Geometry: final body of the model. Coordinates: model frame, mm. Face numbers are marked on the shaded views. A direction names the side the tool comes from. Coordinates: 2 decimals unless noted, no trailing zeros. Write each loop counter-clockwise with the first axis right and the second up, starting at its lowest first coordinate (ties: lowest second). Pieces come first, ordered by that corner, then holes. Notation, with made-up numbers: M 60.25,29 L 68.25,29 A16 ccw 68.25,42 Z; hole C 22,81 d9. An arc over 180 degrees is marked long. Write item = value, one per line. Start each with the question number.
Item 1: First-contact query: pin 1 Ø5 at (y, z) = (6.5, 10.5) entering from +X; pin 2 Ø0.9 at (y, z) = (6.5, 13) entering from +X; pin 3 Ø3 at (y, z) = (5.5, 13.5) entering from -X. Flat tips, straight axial feed; report the tip coordinate or a pass-through.
Item 2: Section A-A on x = 0. Output: boundary loops of the cut face in (y, z).
Item 3: Section D-D on x = -6. Output: boundary loops of the cut face in (y, z).
Item 4: Reachability of the marked faces 5, 6, 7 and 8 from +Z, -Z, +X, -X, +Y, -Y: full face, straight path, thin tool, end or side. Return the list, or none.
Item 5: Ray query, L1, parallel to Z at x = 0, y = 3.5; L2, parallel to X at y = 1.25, z = -10; L3, parallel to X at y = 4.75, z = 6.75. Return the intervals inside material, ascending. Write a range as [from, to].
Item 6: Pull-direction query (Z, two-part tool) for the marked faces 1, 2, 3 and 4; classes: +Z half, -Z half, draft (parallel to the pull), parting line (faces both ways), or undercut.
Item 7: Section B-B on z = 13.25. Output: boundary loops of the cut face in (x, y).
Item 8: Section C-C on z = -5. Output: boundary loops of the cut face in (x, y), plus the area to 3 significant figures.
Autodesk Inventor part; units mm, degrees
ref_plane "Work Plane1" through (0, 10, 0) normal (0, 1, 0) x (-1, 0, 0)
ref_plane "XY Plane" through (0, 0, 0) normal (0, 0, 1) x (1, 0, 0)
sketch "Sketch1" plane through (0, 0, 0) normal (0, 1, 0) x (-1, 0, 0)
  circle A0 centre (0, 0) radius 15
  dimension "d0" = 30
ref_plane "Work Plane1" through (0, 10, 0) normal (0, 1, 0) x (-1, 0, 0)
extrude "Extrusion1" add sketch "Sketch1" along normal blind 10
sketch "Sketch2" plane through (0, 10, 0) normal (0, 1, 0) x (1, 0, 0)
  line L0 (2, -22) -> (-2, -22)
  line L1 (-2, -22) -> (-2, -12)
  line L2 (-2, -12) -> (2, -12)
  line L3 (2, -12) -> (2, -22)
  circle A0 centre (0, 0) radius 15
  point P0 (0, -12)
  dimension "d4" = 4
  dimension "d5" = 10
  dimension "d6" = 12
extrude "Extrusion2" cut sketch "Sketch2" against normal blind 10 contours L0 L1 A0 L3 | A0 L1 L2 L3 picked at (-0.2228, -12.995)
pattern_circular "Circular Pattern1" count 15 over 360 about axis through (0, 0, 0) along (0, 1, 0) of "Extrusion2"
sketch "Sketch6" plane through (0, 10, 0) normal (0, 1, 0) x (1, 0, 0)
  circle A0 centre (0, 0) radius 2.5
  dimension "d24" = 5
extrude "Extrusion6" cut sketch "Sketch6" against normal blind 10
chamfer "Chamfer1" distance 1 angle 45 1 edges at (-2.5, 0, 0)
properties part number "malare" material "Aluminum 6061"
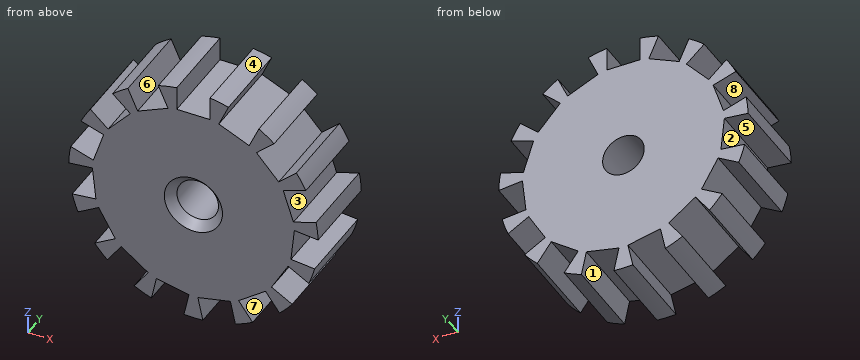
Responses:
q1.pin_1 = 12.69
q1.pin_2 = 8.22
q1.pin_3 = -9
q2.outline = M 0,-15 L 10,-15 L 10,-2.5 L 1,-2.5 L 0,-3.5 Z; M 0,3.5 L 1,2.5 L 10,2.5 L 10,12 L 0,12 Z
q3.outline = M 0,-13.75 L 10,-13.75 L 10,-11.66 L 0,-11.66 Z; M 0,-10.47 L 10,-10.47 L 10,10.46 L 0,10.46 Z
q4.face_5 = +Y, -Y
q4.face_6 = +Z, +Y, -Y
q4.face_7 = +X, +Y, -Y
q4.face_8 = -X, +Y, -Y
q5.L1 = [-15, -2.5], [2.5, 12]
q5.L2 = [-11.18, -9.74], [-6.65, 6.65], [9.74, 11.18]
q5.L3 = [-13.4, -10.49], [-10.07, 10.07], [10.49, 13.4]
q6.face_1 = -Z half
q6.face_2 = undercut
q6.face_3 = undercut
q6.face_4 = +Z half
q7.outline = M -3.71,0 L -2,0 L -2,10 L -3.71,10 Z; M 2,0 L 3.71,0 L 3.71,10 L 2,10 Z
q8.outline = M -14.14,0 L -12.66,0 L -12.66,10 L -14.14,10 Z; M -10.97,0 L 10.97,0 L 10.97,10 L -10.97,10 Z; M 12.66,0 L 14.14,0 L 14.14,10 L 12.66,10 Z
q8.area = 249 mm²
